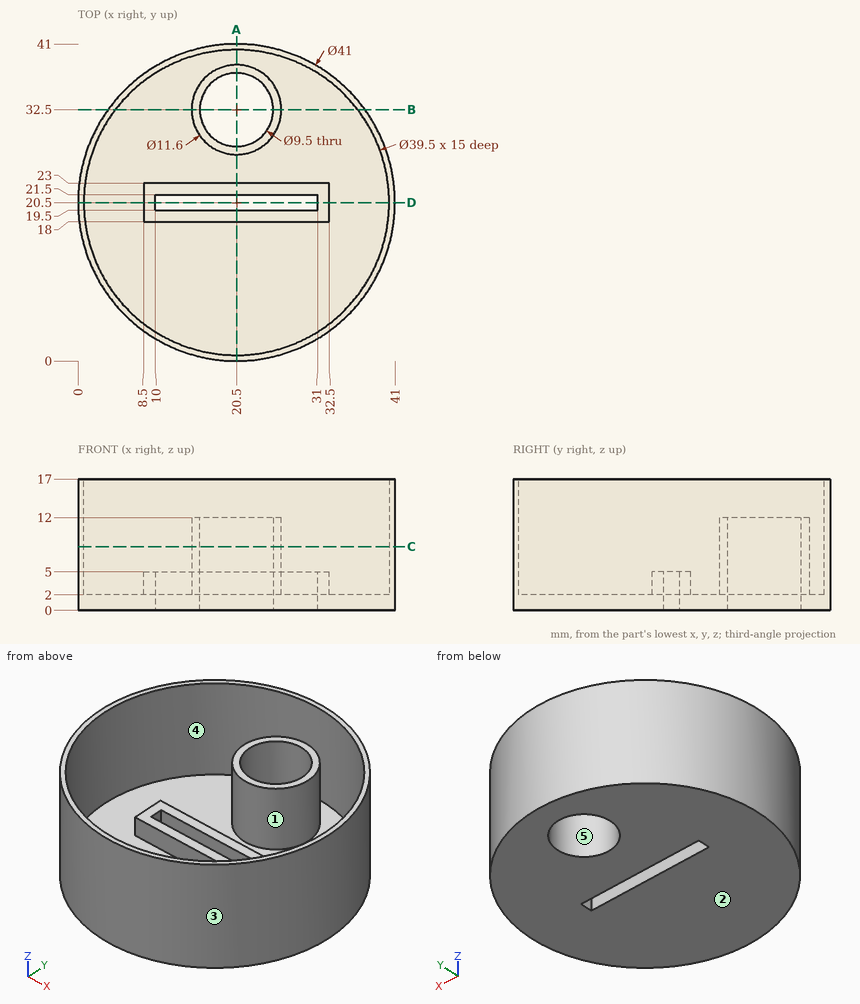
Source: three-view drawing plus pictorial views. Frame: mm from the lowest corner of the part. A direction names the side the tool comes from. Round coordinates to 2 decimals unless told otherwise and drop trailing zeros. Order: outer loops, then holes, each group sorted by start corner. A loop starts at its lowest first (then second) coordinate and runs counter-clockwise, first axis right, second up. Notation, with made-up numbers: (47, 69) - (73, 69) arc R23 cw to (73, 104) - close; hole circle Ø7 at (23.25, -32.75). An arc over 180 degrees is marked (long way). Write each question's results on one line, items separated by ' | '.
Item 1: Reachability of the marked faces 4 and 5 from +Z, -Z, +X, -X, +Y, -Y: full face, straight path, thin tool, end or side. Return the list, or none.
Completed:
face 4: +Z | face 5: +Z, -Z
Item 2: Section C-C, the plane z = 8.25. Return the cut outline in (x, y).
Completed:
outline: circle Ø41 at (20.5, 20.5); circle Ø11.6 at (20.5, 32.5); hole circle Ø39.5 at (20.5, 20.5); hole circle Ø9.5 at (20.5, 32.5)
Item 3: Section B-B, the plane y = 32.5. Return the cut outline in (x, z).
Completed:
outline: (3.88, 0) - (15.75, 0) - (15.75, 12) - (14.7, 12) - (14.7, 2) - (4.81, 2) - (4.81, 17) - (3.88, 17) - close; (25.25, 0) - (37.12, 0) - (37.12, 17) - (36.19, 17) - (36.19, 2) - (26.3, 2) - (26.3, 12) - (25.25, 12) - close
Item 4: First-contact query: pin 1 Ø3 at (y, z) = (23, 7.5) entering from -X; pin 2 Ø12.5 at (x, y) = (20.5, 32.5) entering from -Z; pin 3 Ø5.5 at (x, y) = (15, 20) entering from +Z; pin 4 Ø4 at (x, z) = (24, 9.5) entering from -Y. Flat tips, straight axial feed; report the tip coordinate or a pass-through.
Completed:
pin 1: x = 0.02 | pin 2: z = 0 | pin 3: z = 5 | pin 4: y = 0.05
Item 5: Section D-D, the plane y = 20.5. Return the cut outline in (x, z), and give its area (3 significant figures).
Completed:
outline: (0, 0) - (10, 0) - (10, 5) - (8.5, 5) - (8.5, 2) - (0.75, 2) - (0.75, 17) - (0, 17) - close; (31, 0) - (41, 0) - (41, 17) - (40.25, 17) - (40.25, 2) - (32.5, 2) - (32.5, 5) - (31, 5) - close | area: 71.5 mm^2
Item 6: Mould query, pull axis X, two halves, no side actions, for the marked faces 1, 2 and 3. Classes: pulls with the +X half, pulls with the -X half, needs draft (parallel to the pull), parting line crosses it, or undercut.
Completed:
face 1: undercut | face 2: needs draft | face 3: parting line crosses it
Item 7: Material intervals for line 1 along Y through (x, z) = (20.5, 8); line 2 along X through (y, z) = (36.5, 4.5); line 3 along Y through (x, z) = (24, 9.25), sorted ascending. Write a range as [from, to].
Completed:
line 1: [0, 0.75], [26.7, 27.75], [37.25, 38.3], [40.25, 41] | line 2: [7.68, 8.92], [16.3, 17.94], [23.06, 24.7], [32.08, 33.32] | line 3: [0.3, 1.06], [27.88, 29.29], [35.71, 37.12], [39.94, 40.7]
Item 8: Section A-A, the plane x = 20.5. Return the cut outline in (y, z), and give its area (4 significant figures).
Completed:
outline: (0, 0) - (19.5, 0) - (19.5, 5) - (18, 5) - (18, 2) - (0.75, 2) - (0.75, 17) - (0, 17) - close; (21.5, 0) - (27.75, 0) - (27.75, 12) - (26.7, 12) - (26.7, 2) - (23, 2) - (23, 5) - (21.5, 5) - close; (37.25, 0) - (41, 0) - (41, 17) - (40.25, 17) - (40.25, 2) - (38.3, 2) - (38.3, 12) - (37.25, 12) - close | area: 111.5 mm^2
